from build123d import *

# Parameters (mm, degrees)
EXTRUDE1_DEPTH        = 19.05
F_8_CLEARANCE_HOLE1_D = 4.4958


with BuildPart() as part:
    # Sketch1 → Extrude1 (new body)
    with BuildSketch(Plane.XY):
        Polygon((0, 0), (-38.1, 0), (-38.1, -16.0528), (-52.705, -16.0528), (-52.705, -19.2278), (-34.925, -19.2278), (-34.925, -3.175), (0, -3.175), align=None)
    extrude1 = extrude(amount=EXTRUDE1_DEPTH)

    # #8 Clearance Hole1 (through all)
    with Locations(Plane(origin=(-46.6344, -16.0528, 4.445), x_dir=(1, 0, 0), z_dir=(0, 1, 0))):
        with Locations((0, 0), (0, -10.16)):
            f_8_clearance_hole1 = Hole(F_8_CLEARANCE_HOLE1_D / 2)

    # Mirror1: Extrude1, #8 Clearance Hole1 across plane
    add(extrude1.mirror(Plane(origin=(0, 0, 0), x_dir=(0, 0, 1), z_dir=(1, 0, 0))))
    add(f_8_clearance_hole1.mirror(Plane(origin=(0, 0, 0), x_dir=(0, 0, 1), z_dir=(1, 0, 0))), mode=Mode.SUBTRACT)


solid = part.part
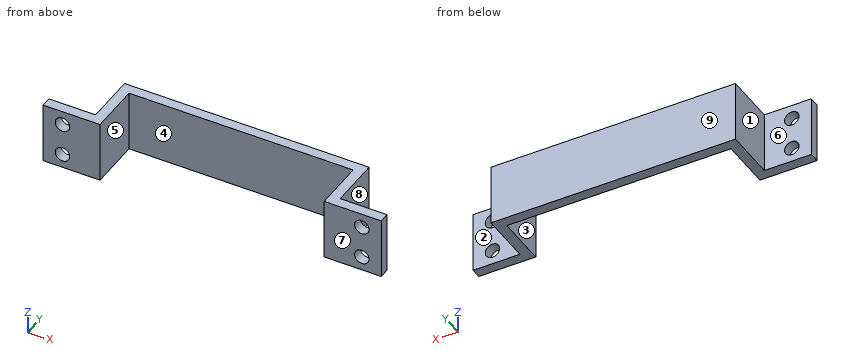
CAD build for the part. Positions are in the model's coordinates, mm. Face numbers are marked on the shaded views. A direction names the side the tool comes from. Round coordinates to 2 decimals unless told otherwise and drop trailing zeros. Write each loop counter-clockwise with the first axis right and the second up, starting at its lowest first coordinate (ties: lowest second). Pieces come first, ordered by that corner, then holes. Notation, with made-up numbers: (19, -30) -> (23, -30) arc R19 ccw to (23, -1) -> close; hole circle Ø5 at (-23, -11.5). An arc over 180 degrees is marked (long way). Answer as a JSON object with one key per item and string values.
(1) Probe probe 1 along X at (y, z) = (-17.5, 4.25) (3 decimals); probe 2 along X at (y, z) = (-8.75, 7.5) (3 decimals); probe 3 along X at (y, z) = (-2.75, 16.75). List the from-to ranges inside material, lowest first. Write a range as [from, to].
Reported:
{"probe 1": "x = [-52.705, -48.874], [-44.395, -34.925], [34.925, 44.395], [48.874, 52.705]", "probe 2": "x = [-38.1, -34.925], [34.925, 38.1]", "probe 3": "x = [-38.1, 38.1]"}
(2) Band-saw the part on C-C, the plane x = 46. List the corners of the cut face in (y, z).
Reported:
{"outline": "(-19.23, 0) -> (-16.05, 0) -> (-16.05, 2.29) -> (-19.23, 2.29) -> close; (-19.23, 6.6) -> (-16.05, 6.6) -> (-16.05, 12.45) -> (-19.23, 12.45) -> close; (-19.23, 16.76) -> (-16.05, 16.76) -> (-16.05, 19.05) -> (-19.23, 19.05) -> close"}
(3) Band-saw the part on A-A, the plane y = -17. List the corners of the cut face in (x, z) (3 decimals).
Reported:
{"outline": "(-52.705, 0) -> (-34.925, 0) -> (-34.925, 19.05) -> (-52.705, 19.05) -> close; (34.925, 0) -> (52.705, 0) -> (52.705, 19.05) -> (34.925, 19.05) -> close; hole circle Ø4.496 at (-46.634, 4.445); hole circle Ø4.496 at (-46.634, 14.605); hole circle Ø4.496 at (46.634, 4.445); hole circle Ø4.496 at (46.634, 14.605)"}
(4) Which spindle directions (+Z, -Z, +X, -X, +Y, -Y) get a long thin tool onto all of the face, cutting with end or side? Do the marked faces 5, 6, 7, 8 and 9. Say none if no direction does.
Reported:
{"face 5": "+Z, -Z, -Y", "face 6": "+Z, -Z, -X, +Y", "face 7": "+Z, -Z, +X, -X, -Y", "face 8": "+Z, -Z, +X, +Y", "face 9": "+Z, -Z, +X, -X, +Y"}
(5) Pin check, flat tips, straight feed: P1, Ø8, axis at x = -15, y = -3.5, coming from the -Z side; P2, Ø7, axis at x = 46.63, z = 4.44, coming from the +Y side; P3, Ø3, axis at y = -7.5, z = 15.5, coming from the +X side; P4, Ø4, axis at y = -7, z = 14, coming from the -X side. Stop position of each tip, or through.
Reported:
{"P1": "stops at z = 0", "P2": "stops at y = -16.05", "P3": "stops at x = 38.1", "P4": "stops at x = -38.1"}
(6) Band-saw the part on B-B, the plane y = -10.25. List the corners of the cut face in (x, z) (3 decimals), then the cut area to 3 significant figures.
Reported:
{"outline": "(-38.1, 0) -> (-34.925, 0) -> (-34.925, 19.05) -> (-38.1, 19.05) -> close; (34.925, 0) -> (38.1, 0) -> (38.1, 19.05) -> (34.925, 19.05) -> close", "area": "121 mm^2"}
(7) Two-plate mould, pull along X, no slides. Class the marked faces 1, 2, 3 and 4: +X half, -X half, draft (parallel to the pull), parting line (faces both ways), or undercut.
Reported:
{"face 1": "-X half", "face 2": "draft", "face 3": "undercut", "face 4": "undercut"}
(8) Band-saw the part on D-D, the plane z = 13.5. List the corners of the cut face in (x, y) (3 decimals).
Reported:
{"outline": "(-52.705, -19.228) -> (-48.592, -19.228) -> (-48.592, -16.053) -> (-52.705, -16.053) -> close; (-44.677, -19.228) -> (-34.925, -19.228) -> (-34.925, -3.175) -> (34.925, -3.175) -> (34.925, -19.228) -> (44.677, -19.228) -> (44.677, -16.053) -> (38.1, -16.053) -> (38.1, 0) -> (-38.1, 0) -> (-38.1, -16.053) -> (-44.677, -16.053) -> close; (48.592, -19.228) -> (52.705, -19.228) -> (52.705, -16.053) -> (48.592, -16.053) -> close"}
